Model file for the job. Use its own axes, mm. Face numbers are marked on the shaded views. A direction names the side the tool comes from. Give positions to 0.01 mm unless a question says otherwise; leave off trailing zeros. Loops run counter-clockwise (first coordinate to the right, second up) from the corner with the lowest first, then second, coordinate; pieces in that order, holes last. Notation, with made-up numbers: M 44,52 L 64,52 A14 ccw 64,63 Z; hole C 67,-39 d7. An arc over 180 degrees is marked long. Answer in a Markdown table with one row per item.
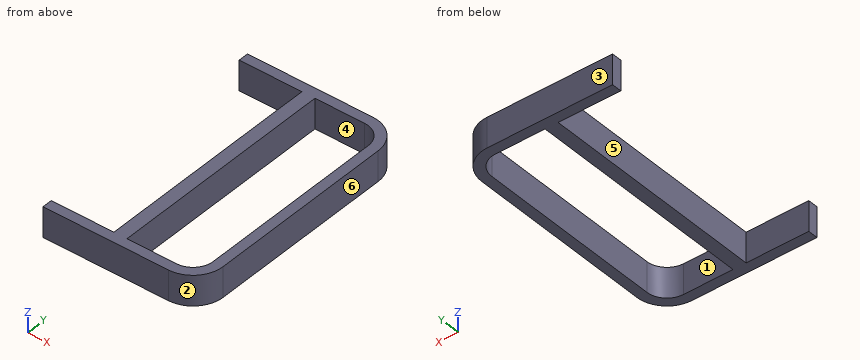
```python
from build123d import *

# Parameters (mm, degrees)
SKETCH2_W           = 152.4
SKETCH2_H           = 50.8
SKETCH3_W           = 66.098972621
SKETCH3_H           = 152.4
BOSS_EXTRUDE1_DEPTH = 1229.106


with BuildPart() as part:
    # Sweep1: sweep along a path in Sketch1
    with BuildLine(Plane.XY) as sweep1_path:
        Line((0, 0), (635, 0))
        ThreePointArc((635, 0), (724.802561211, -37.197438789), (762, -127))
        Line((762, -127), (762, -1083.056))
        ThreePointArc((762, -1083.056), (724.802561211, -1172.858561211), (635, -1210.056))
        Line((635, -1210.056), (0, -1210.056))
    # Sketch2 → Sweep1 (sweep)
    with BuildSketch(Plane(origin=(0, 0, 0), x_dir=(0, 0, -1), z_dir=(1, 0, 0))):
        Rectangle(SKETCH2_W, SKETCH2_H)
    sweep(path=sweep1_path.line)

    # Sketch3 → Boss-Extrude1 (add)
    with BuildSketch(Plane(origin=(0, 25.4, 0), x_dir=(1, 0, 0), z_dir=(0, 1, 0))):
        with Locations((350.549486311, 0)):
            Rectangle(SKETCH3_W, SKETCH3_H)
    extrude(amount=-BOSS_EXTRUDE1_DEPTH)


solid = part.part
```
Q1. 3-axis set-ups, long thin cutter, end or side, ignore diameter. For the marked faces 4, 5 and 6: which of +Z, -Z, +X, -X, +Y, -Y reach the whole face in a straight line?
Reported:
| item | result |
|---|---|
| face 4 | +Z, -Z |
| face 5 | +Z, -Z, -X |
| face 6 | +Z, -Z, +X, +Y, -Y |
Q2. Probe probe 1 along X at (y, z) = (-529.5, 9); probe 2 along Y at (x, z) = (105, 38); probe 3 along X at (y, z) = (-109, 46.5). List the from-to ranges inside material, lowest first.
Reported:
| item | result |
|---|---|
| probe 1 | 317.5 to 383.6, 736.6 to 787.4 |
| probe 2 | -1235.46 to -1184.66, -25.4 to 25.4 |
| probe 3 | 317.5 to 383.6, 734.99 to 786.33 |
Q3. Saw through at A-A (y = -289.5). Give the cut face in (x, z).
Reported:
| item | result |
|---|---|
| outline | M 317.5,-76.2 L 383.6,-76.2 L 383.6,76.2 L 317.5,76.2 Z; M 736.6,-76.2 L 787.4,-76.2 L 787.4,76.2 L 736.6,76.2 Z |
Q4. Mould opens along Y. For the marked faces 1, 2 and 3 say: released by +Y, released by -Y, zero draft, split by the parting line, or undercut.
Reported:
| item | result |
|---|---|
| face 1 | undercut |
| face 2 | released by -Y |
| face 3 | released by +Y |
Q5. Drop a flat-ended pin along its axis: pin 1 (10 mm diameter, centred on x = 645.5, z = -12.5, fed in from -Y). Give the stop position or say it passes through.
Reported:
| item | result |
|---|---|
| pin 1 | y = -1235.36 |
Q6. Saw through at C-C (z = 7). Give the cut face in (x, y).
Reported:
| item | result |
|---|---|
| outline | M 0,-1235.46 L 635,-1235.46 A152.4 ccw 787.4,-1083.06 L 787.4,-127 A152.4 ccw 635,25.4 L 0,25.4 L 0,-25.4 L 317.5,-25.4 L 317.5,-1184.66 L 0,-1184.66 Z; hole M 383.6,-1184.66 L 635,-1184.66 A101.6 ccw 736.6,-1083.06 L 736.6,-127 A101.6 ccw 635,-25.4 L 383.6,-25.4 Z |
Q7. Saw through at B-B (x = 189.5). Give the cut face in (y, z).
Reported:
| item | result |
|---|---|
| outline | M -1235.46,-76.2 L -1184.66,-76.2 L -1184.66,76.2 L -1235.46,76.2 Z; M -25.4,-76.2 L 25.4,-76.2 L 25.4,76.2 L -25.4,76.2 Z |
